The drawing under review shows one solid part. Ordinate dimensions are in mm from its lowest x, y, z. A direction names the side the tool comes from. Round coordinates to 2 decimals unless told otherwise and drop trailing zeros. Order: outer loops, then holes, each group sorted by start corner. A loop starts at its lowest first (then second) coordinate and runs counter-clockwise, first axis right, second up.
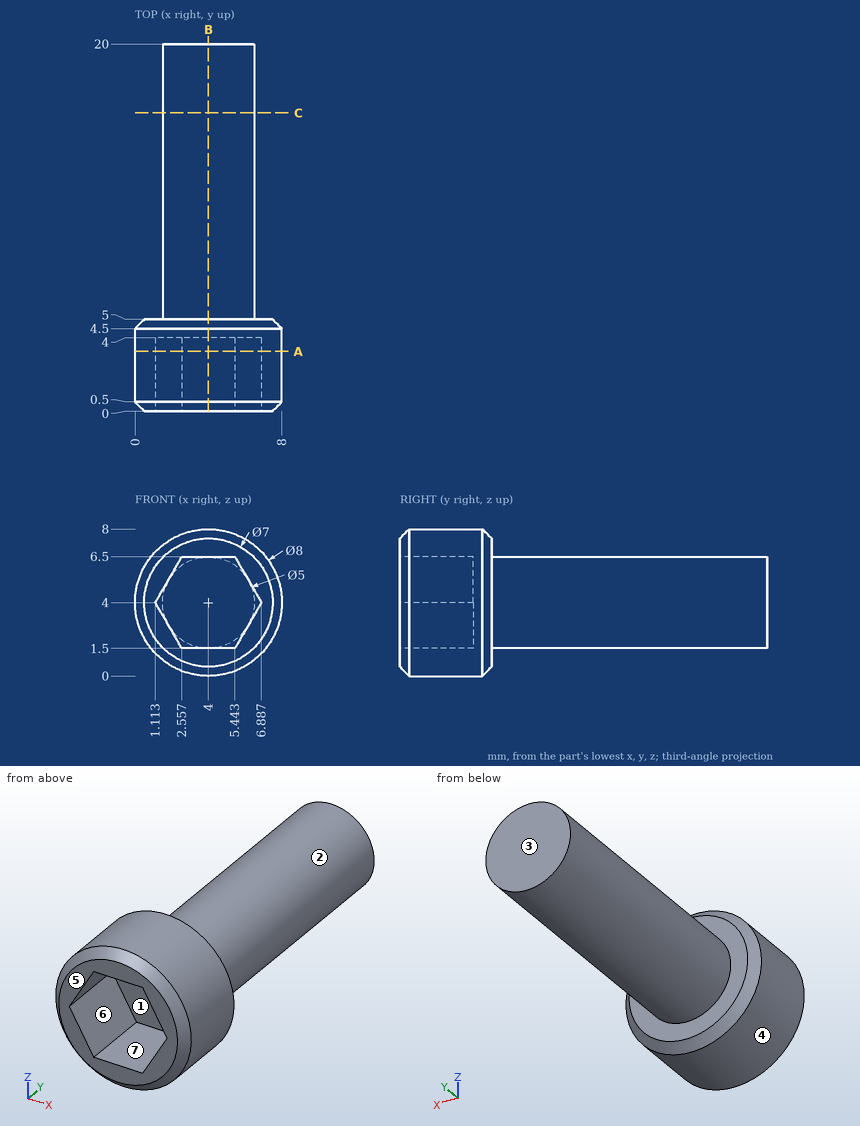
Q1. Mouldability with a two-part tool opening along X and no side actions: class the marked faces 4, 5, 6 and 7 as +X half, -X half, draft (parallel to the pull), parting line (faces both ways), or undercut.
Q2. Take a section at C-C, the plane y = 16.25. State the section outline as (x, z) points, plus the area to 3 significant figures.
Q3. Tool access review of the marked faces 1, 2 and 3: name each direction out of +Z, -Z, +X, -X, +Y, -Y from which nothing blocks a thin tool from reaching the whole face with its end or side.
Q4. Wall thickness on line 1 (Y direction, x = 5.25, z = 3.75); line 2 (Z direction, x = 5.75, y = 2.5) (1 decimal); line 3 (Z direction, x = 5.25, y = 2.5): over which ranges is each line inside the solid? List them lowest first.
Q5. Take a section at B-B, the plane x = 4. State the section outline as (y, z) points.
Q6. Take a section at A-A, the plane y = 3.25. State the section outline as (x, z) points.
Q7. Clearance check with flat-ended pins moving along their axes: pin 1 (3 mm diameter, centred on x = 5.5, y = 17.5, fed in from -Z); pin 2 (1.5 mm diameter, centred on y = 7.5, z = 3, fed in from -X); pin 3 (1.5 mm diameter, centred on x = 7, y = 5.5, fed in from +Z). State where each tip first meets the part, or that it passes through.
Working result:
1. face 4: parting line
1. face 5: draft
1. face 6: undercut
1. face 7: undercut
2. outline: circle Ø5 at (4, 4)
2. area: 19.6 mm2
3. face 1: -Y
3. face 2: +Y
3. face 3: +Z, -Z, +X, -X, +Y
4. line 1: y = 4 to 20
4. line 2: z = 0.4 to 2, 6 to 7.6
4. line 3: z = 0.2 to 1.5, 6.5 to 7.8
5. outline: (0, 0.5) - (0.5, 0) - (4.5, 0) - (5, 0.5) - (5, 1.5) - (20, 1.5) - (20, 6.5) - (5, 6.5) - (5, 7.5) - (4.5, 8) - (0.5, 8) - (0, 7.5) - (0, 6.5) - (4, 6.5) - (4, 1.5) - (0, 1.5) - close
6. outline: circle Ø8 at (4, 4); hole (1.11, 4) - (2.56, 1.5) - (5.44, 1.5) - (6.89, 4) - (5.44, 6.5) - (2.56, 6.5) - close
7. pin 1: stops at z = 1.5
7. pin 2: stops at x = 1.51
7. pin 3: stops at z = 6.54
